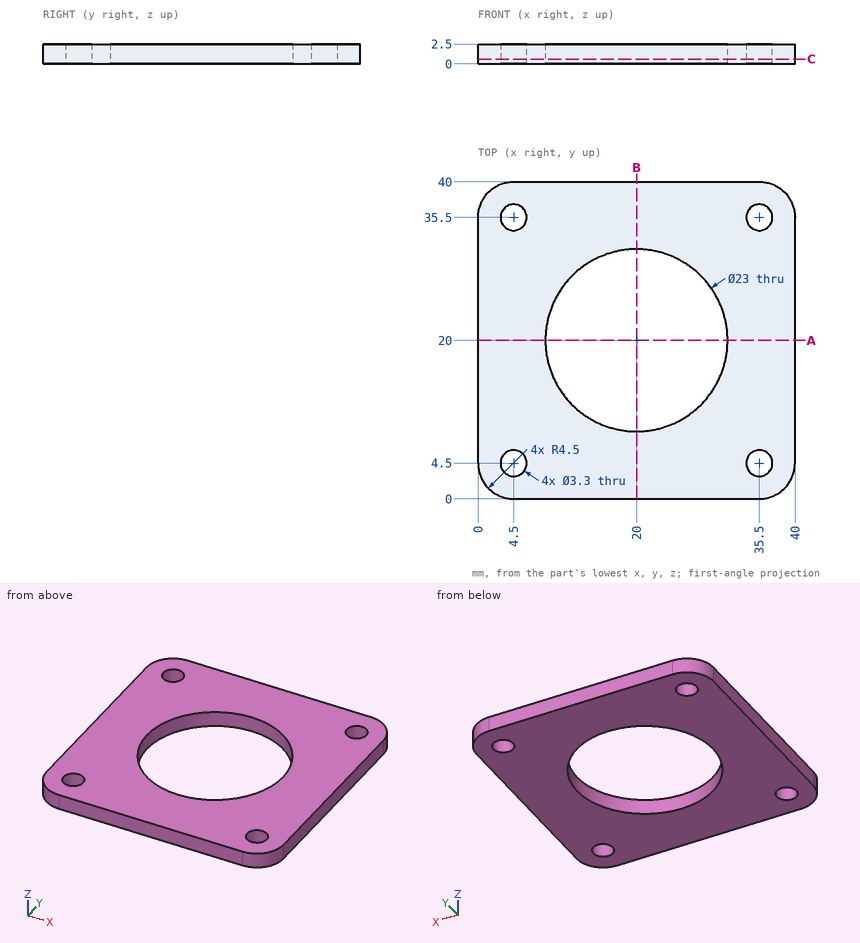
Job drawing, mm, ordinate dimensions from the low corner. One solid piece. Coordinates: 2 decimals unless noted, no trailing zeros. Order: outer loops, then holes, each group sorted by start corner. A loop starts at its lowest first (then second) coordinate and runs counter-clockwise, first axis right, second up. Notation, with made-up numbers: (-10, 11) -> (41, 11) arc R15 ccw to (41, 20) -> close; hole circle Ø8 at (58, -20.75). An arc over 180 degrees is marked (long way). Return JSON: item names as keys, results as strings. Group by question number.
Item 1: Saw through at A-A on y = 20. Write the cut outline in (x, z).
Item 2: Saw through at C-C on z = 0.6. Write the cut outline in (x, y), then the cut area to 3 significant figures.
Item 3: Wall check: line 1 along Y through (x, z) = (35.5, 1.85); line 2 along Y through (x, z) = (20, 0.8); line 3 along X through (y, z) = (17.5, 1.15). Give the ranges that are in metal, low to high. Write a range as [from, to].
Values found:
{
 "1": {"outline": "(0, 0) -> (8.5, 0) -> (8.5, 2.5) -> (0, 2.5) -> close; (31.5, 0) -> (40, 0) -> (40, 2.5) -> (31.5, 2.5) -> close"},
 "2": {"outline": "(0, 4.5) arc R4.5 ccw to (4.5, 0) -> (35.5, 0) arc R4.5 ccw to (40, 4.5) -> (40, 35.5) arc R4.5 ccw to (35.5, 40) -> (4.5, 40) arc R4.5 ccw to (0, 35.5) -> close; hole circle Ø3.3 at (4.5, 4.5); hole circle Ø3.3 at (4.5, 35.5); hole circle Ø23 at (20, 20); hole circle Ø3.3 at (35.5, 4.5); hole circle Ø3.3 at (35.5, 35.5)", "area": "1,130 mm2"},
 "3": {"line 1": "y = [0, 2.85], [6.15, 33.85], [37.15, 40]", "line 2": "y = [0, 8.5], [31.5, 40]", "line 3": "x = [0, 8.78], [31.22, 40]"}
}
